```python
from build123d import *

# Parameters (mm, degrees)
SKETCH1_R           = 1.7859375
BOSS_EXTRUDE1_DEPTH = 1.5875
FILLET1_R           = 3.571875


with BuildPart() as part:
    # Sketch1 → Boss-Extrude1 (new body)
    with BuildSketch(Plane.XY):
        with BuildLine():
            ThreePointArc((25.4, -12.7), (28.971875, -9.128125), (25.4, -5.55625))
            ThreePointArc((25.4, -5.55625), (30.95625, 0), (25.4, 5.55625))
            Line((25.4, 5.55625), (19.614019559, 5.55625))
            ThreePointArc((19.614019559, 5.55625), (16.929229109, 11.484009389), (14.244438658, 5.55625))
            Line((14.244438658, 5.55625), (0.813693974, 5.55625))
            ThreePointArc((0.813693974, 5.55625), (0.238325447, 5.317924553), (0, 4.742556026))
            Line((0, 4.742556026), (0, 2.778125))
            ThreePointArc((0, 2.778125), (0.813693974, 0.813693974), (2.778125, 0))
            Line((2.778125, 0), (12.7, 0))
            ThreePointArc((12.7, 0), (16.419743879, -8.980256121), (25.4, -12.7))
        make_face()
        with BuildLine():
            ThreePointArc((18.08575174, 0.639913805), (19.986771554, -4.960309977), (25.4, -7.3421875))
            ThreePointArc((25.4, -7.3421875), (27.1859375, -9.128125), (25.4, -10.9140625))
            ThreePointArc((25.4, -10.9140625), (17.353309066, -7.37343375), (14.527468803, 0.951223224))
            ThreePointArc((14.527468803, 0.951223224), (16.462264981, 2.574709983), (18.08575174, 0.639913805))
        make_face(mode=Mode.SUBTRACT)
        with Locations((25.4, 0)):
            Circle(SKETCH1_R, mode=Mode.SUBTRACT)
        with Locations((16.929229109, 7.912134389)):
            Circle(SKETCH1_R, mode=Mode.SUBTRACT)
    extrude(amount=BOSS_EXTRUDE1_DEPTH)

    # Fillet1
    fillet1_edges = [part.edges().sort_by_distance(p)[0] for p in [
        (14.244438658, 5.55625, 0.79375),
        (19.614019559, 5.55625, 0.79375),
        (25.4, -5.55625, 0.79375),
        (12.7, 0, 0.79375),
    ]]
    fillet(fillet1_edges, radius=FILLET1_R)


solid = part.part
```
Geometry check sheet. Reference: the model listing, model coordinates, mm. A direction names the side the tool comes from. Coordinates: 2 decimals unless noted, no trailing zeros. Order: outer loops, then holes, each group sorted by start corner. A loop starts at its lowest first (then second) coordinate and runs counter-clockwise, first axis right, second up.
Q1. Tool access check on faces 1 (the face through (6, 0, 1)), 2 (the face through (19.93, -4.9, 0.78)), 3 (the face through (5, 5.556, 1)). Record the directions out of +Z, -Z, +X, -X, +Y, -Y that give a thin tool (end or side, any length) a straight path to the whole face; none if there is none.
Reply:
face 1: +Z, -Z, -X, -Y
face 2: +Z, -Z
face 3: +Z, -Z, -X, +Y
Q2. Draft check along Y on faces 4 (the face through (25, 5.556, 1)), 5 (the face through (16.54, 6.17, 0.78)), 6 (the face through (11.78, -0.8, 0.8)). Enter one of: released by +Y, released by -Y, zero draft, split by the parting line, or undercut.
Reply:
face 4: released by +Y
face 5: undercut
face 6: released by -Y
Q3. Sectioned sample at C-C on y = -2.25. Record the cut outline in (x, z), and give its area (3 significant figures).
Reply:
outline: (12.84, 0) - (14.72, 0) - (14.72, 1.59) - (12.84, 1.59) - close; (18.41, 0) - (30.48, 0) - (30.48, 1.59) - (18.41, 1.59) - close
area: 22.1 mm2
Q4. Sectioned sample at A-A on y = 9. Record the cut outline in (x, z).
Reply:
outline: (13.53, 0) - (15.51, 0) - (15.51, 1.59) - (13.53, 1.59) - close; (18.35, 0) - (20.33, 0) - (20.33, 1.59) - (18.35, 1.59) - close
Q5. Thickness scan on probe 1 along Y at (x, z) = (25.4, 0.55); probe 2 along Y at (x, z) = (27, 0.95); probe 3 along X at (y, z) = (1, 1.3). Record the ranges inside material, lowest first.
Reply:
probe 1: y = -12.7 to -10.91, -7.34 to -1.79, 1.79 to 5.56
probe 2: y = -12.32 to -9.92, -8.33 to -0.79, 0.79 to 5.32
probe 3: x = 0.64 to 14.53, 18.08 to 23.92, 26.88 to 30.87
Q6. Sectioned sample at B-B on x = 26.5. Record the cut outline in (y, z).
Reply:
outline: (-12.53, 0) - (-10.54, 0) - (-10.54, 1.59) - (-12.53, 1.59) - close; (-7.72, 0) - (-1.41, 0) - (-1.41, 1.59) - (-7.72, 1.59) - close; (1.41, 0) - (5.45, 0) - (5.45, 1.59) - (1.41, 1.59) - close
Q7. Sectioned sample at D-D on x = 9. Record the cut outline in (y, z).
Reply:
outline: (0, 0) - (5.56, 0) - (5.56, 1.59) - (0, 1.59) - close
